For this review, use the dimensioned drawing (mm, ordinates from the lowest corner) and the shaded views. A direction names the side the tool comes from. Round coordinates to 2 decimals unless told otherwise and drop trailing zeros. Order: outer loops, then holes, each group sorted by start corner. A loop starts at its lowest first (then second) coordinate and runs counter-clockwise, first axis right, second up. Notation, with made-up numbers: (28, 76) -> (83, 76) arc R19 ccw to (83, 98) -> close; hole circle Ø4 at (38, 64.5). An arc over 180 degrees is marked (long way). Answer in a Markdown table with one row per item.
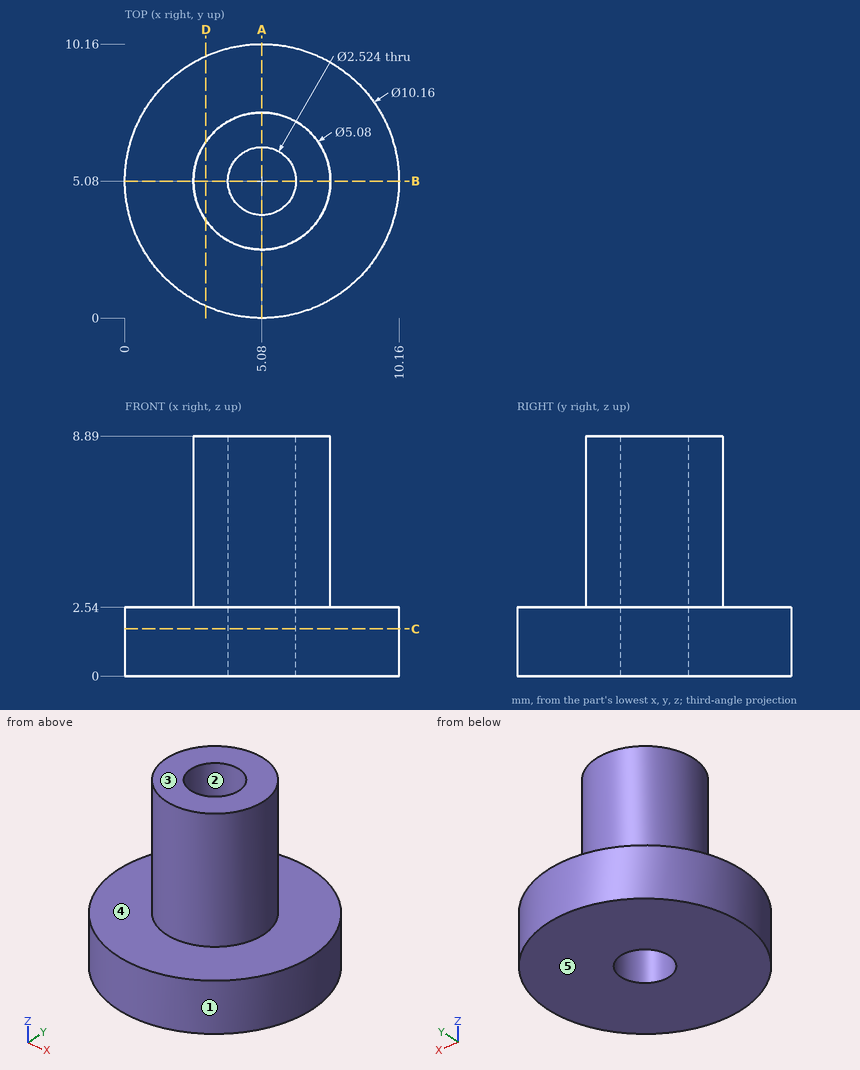
Q1. Take a section at C-C, the plane z = 1.75. Write out the cut boundary in (x, y).
Answer key:
| item | result |
|---|---|
| outline | circle Ø10.16 at (5.08, 5.08); hole circle Ø2.52 at (5.08, 5.08) |
Q2. To check wall thickness, follow probe 1 along X at (y, z) = (5.08, 6.25); probe 2 along Y at (x, z) = (5, 1.5). State the ranges of each line that lie inside material, in increasing order.
Answer key:
| item | result |
|---|---|
| probe 1 | x = 2.54 to 3.82, 6.34 to 7.62 |
| probe 2 | y = 0 to 3.82, 6.34 to 10.16 |
Q3. Clearance check with flat-ended pins moving along their axes: pin 1 Ø1.5 at (x, y) = (5.08, 5.08) entering from +Z; pin 2 Ø1.5 at (x, z) = (6.5, 1.5) entering from -Y; pin 3 Ø2 at (x, z) = (5.5, 5.5) entering from -Y. State where each tip first meets the part, or that it passes through.
Answer key:
| item | result |
|---|---|
| pin 1 | passes through |
| pin 2 | stops at y = 0.04 |
| pin 3 | stops at y = 2.54 |
Q4. The part is to be moulded in two halves that separate along Y. For the marked faces 1, 2 and 3, say which applies: +Y half, -Y half, draft (parallel to the pull), parting line (faces both ways), or undercut.
Answer key:
| item | result |
|---|---|
| face 1 | parting line |
| face 2 | undercut |
| face 3 | draft |
Q5. Tool access review of the marked faces 4 and 5: name each direction out of +Z, -Z, +X, -X, +Y, -Y from which nothing blocks a thin tool from reaching the whole face with its end or side.
Answer key:
| item | result |
|---|---|
| face 4 | +Z |
| face 5 | -Z, +X, -X, +Y, -Y |
Q6. Take a section at D-D, the plane x = 3. Write out the cut boundary in (y, z) (1 decimal).
Answer key:
| item | result |
|---|---|
| outline | (0.4, 0) -> (9.7, 0) -> (9.7, 2.5) -> (6.5, 2.5) -> (6.5, 8.9) -> (3.6, 8.9) -> (3.6, 2.5) -> (0.4, 2.5) -> close |
Q7. Take a section at A-A, the plane x = 5.08. Write out the cut boundary in (y, z), then the cut area to 3 significant figures.
Answer key:
| item | result |
|---|---|
| outline | (0, 0) -> (3.82, 0) -> (3.82, 8.89) -> (2.54, 8.89) -> (2.54, 2.54) -> (0, 2.54) -> close; (6.34, 0) -> (10.16, 0) -> (10.16, 2.54) -> (7.62, 2.54) -> (7.62, 8.89) -> (6.34, 8.89) -> close |
| area | 35.6 mm^2 |
